Check sheet for the modelled part. Datum: model origin and axes. Units: mm. Coordinates: 2 decimals unless noted, no trailing zeros. Loops run counter-clockwise (first coordinate to the right, second up) from the corner with the lowest first, then second, coordinate; pieces in that order, holes last.
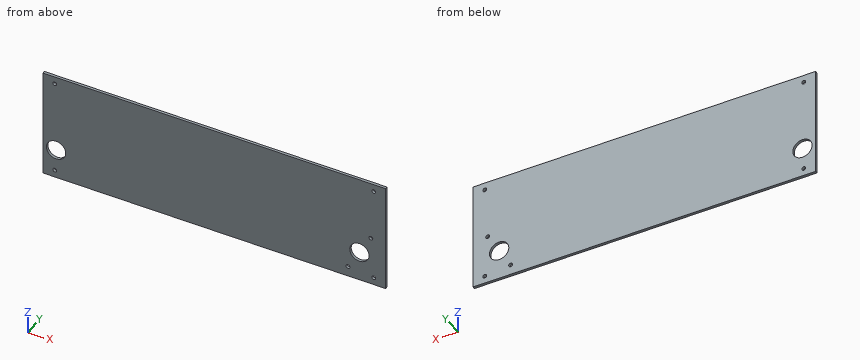
```python
from build123d import *

# Parameters (mm, degrees)
SKETCH_1_W         = 262.1
SKETCH_1_H         = 84
EXTRUDE_1_DEPTH    = 1
SKETCH1_R          = 1.5
CUT_EXTRUDE1_DEPTH = 10
SKETCH4_R          = 7.4
CUT_EXTRUDE3_DEPTH = 138.630310978
SKETCH5_R          = 1.5
CUT_EXTRUDE4_DEPTH = 10


with BuildPart() as part:
    # 草图1 → 凸台-拉伸1 (new, symmetric)
    with BuildSketch(Plane(origin=(0, 0, 0), x_dir=(1, 0, 0), z_dir=(0, 1, 0))):
        Rectangle(SKETCH_1_W, SKETCH_1_H)
    extrude(amount=EXTRUDE_1_DEPTH, both=True)

    # Sketch1 → Cut-Extrude1 (cut)
    with BuildSketch(Plane(origin=(0, 1, 0), x_dir=(1, 0, 0), z_dir=(0, 1, 0))):
        with Locations(Location((-122.05, 36.25, 0), (0, 0, 270))):
            Circle(SKETCH1_R)
        with Locations(Location((-122.05, -36.25, 0), (0, 0, 270))):
            Circle(SKETCH1_R)
        with Locations(Location((122.05, -36.25, 0), (0, 0, 270))):
            Circle(SKETCH1_R)
        with Locations(Location((122.05, 36.25, 0), (0, 0, 270))):
            Circle(SKETCH1_R)
    extrude(amount=-CUT_EXTRUDE1_DEPTH, mode=Mode.SUBTRACT)

    # Sketch4 → Cut-Extrude3 (cut, through all)
    with BuildSketch(Plane(origin=(0, 1, 0), x_dir=(1, 0, 0), z_dir=(0, 1, 0))):
        with Locations(Location((-121.050000944, 19, 0), (0, 0, 270))):
            Circle(SKETCH4_R)
        with Locations(Location((111.049999056, 19, 0), (0, 0, 270))):
            Circle(SKETCH4_R)
    extrude(amount=-CUT_EXTRUDE3_DEPTH, mode=Mode.SUBTRACT)

    # Sketch5 → Cut-Extrude4 (cut)
    with BuildSketch(Plane(origin=(0, 1, 0), x_dir=(1, 0, 0), z_dir=(0, 1, 0))):
        with Locations(Location((119.799998238, 3.844554962, 0), (0, 0, 270))):
            Circle(SKETCH5_R)
        with Locations(Location((102.299999873, 34.155445038, 0), (0, 0, 270))):
            Circle(SKETCH5_R)
    extrude(amount=-CUT_EXTRUDE4_DEPTH, mode=Mode.SUBTRACT)


solid = part.part
```
1) Section check C-C on x = 111.05. Enter the section's corners in (y, z).
Answer sheet:
outline: (-1, -42) - (1, -42) - (1, -26.4) - (-1, -26.4) - close; (-1, -11.6) - (1, -11.6) - (1, 42) - (-1, 42) - close
2) Scan lines: line 1 (Z direction, x = 122.05, y = -0.05); line 2 (Z direction, x = 102, y = 0.1); line 3 (Z direction, x = -122.05, y = 0.05). Record each from-to range of solid material in increasing order.
Answer sheet:
line 1: z = -42 to -37.75, -34.75 to 34.75, 37.75 to 42
line 2: z = -42 to -35.63, -32.69 to 42
line 3: z = -42 to -37.75, -34.75 to -26.33, -11.67 to 34.75, 37.75 to 42
3) Section check A-A on y = 0.3. Give the number of separate pieces and of enclosed holes in the cut face, plus the area to 3 significant figures.
Answer sheet:
separate pieces: 1
enclosed holes: 8
area: 21,600 mm2
4) Section check B-B on z = -19. Enter the section's corners in (x, y), plus the area to 3 significant figures.
Answer sheet:
outline: (-131.05, -1) - (-128.45, -1) - (-128.45, 1) - (-131.05, 1) - close; (-113.65, -1) - (103.65, -1) - (103.65, 1) - (-113.65, 1) - close; (118.45, -1) - (131.05, -1) - (131.05, 1) - (118.45, 1) - close
area: 465 mm2
5) Depth check by flat-ended pin: pin 1 (2.5 mm diameter, centred on x = -122.05, z = 36.25, fed in from +Y). Enter the tip coordinate at first touch or a pass-through.
Answer sheet:
pin 1: passes through
